Study the drawing (mm; zero at the part's minimum x, y, z) and answer. A direction names the side the tool comes from. Coordinates: 2 decimals unless noted, no trailing zeros. Order: outer loops, then holes, each group sorted by start corner. A loop starts at its lowest first (then second) coordinate and runs counter-clockwise, first axis right, second up. Notation, with made-up numbers: (62.25, -20.5) -> (108.25, -20.5) arc R29 ccw to (108.25, 15.5) -> close; hole circle Ø7 at (16, 29.5). An arc over 180 degrees is marked (long way). Put each result on its own line as item: value. Start each with the question number.
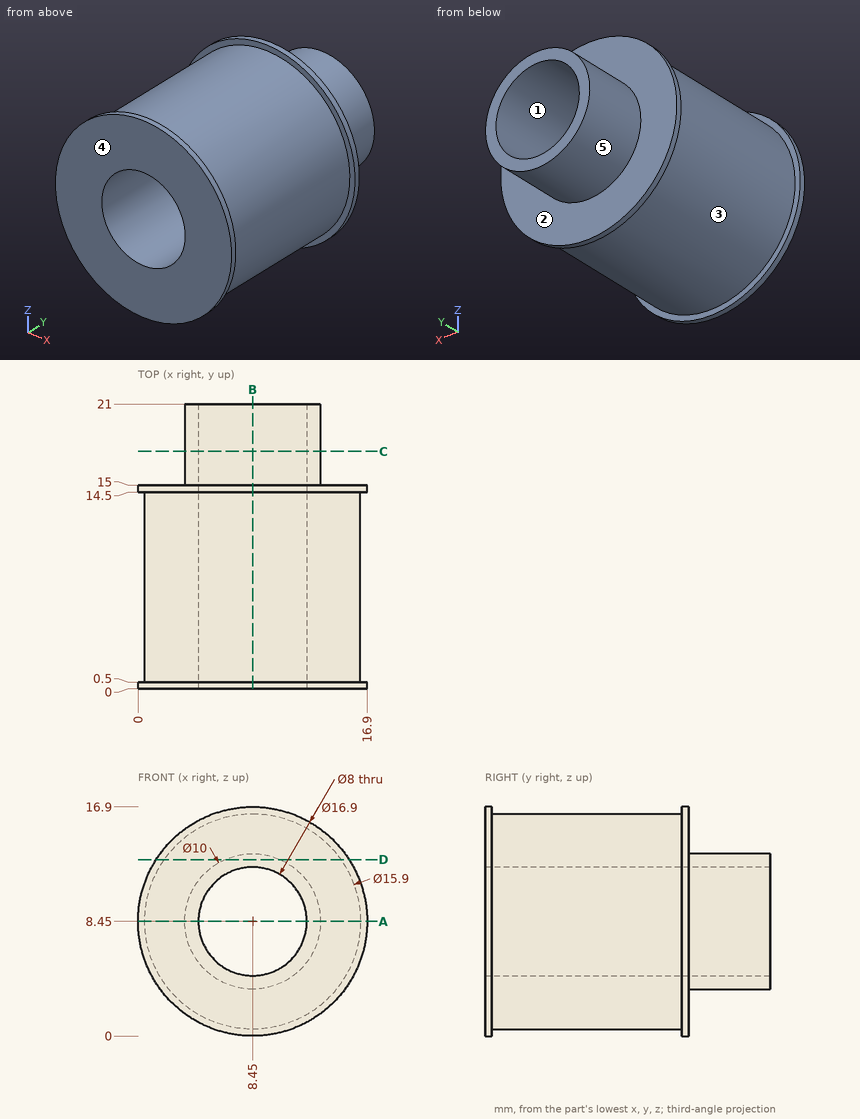
(1) The part is cut by section A-A on z = 8.45. Determine the outline of the cut face in (x, y).
(2) A tool of negligible diameter and unlimited length cuts with its end or side. For the marked faces 4 and 5, from which of +Z, -Z, +X, -X, +Y, -Y can it reach the whole face along a straight path? Write none if from no direction.
(3) For a pull along X with two mould halves and no side action, classify the marked faces 1, 2 and 3 as released by +X, released by -X, zero draft, split by the parting line, or undercut.
(4) The part is cut by section C-C on y = 17.5. Determine the outline of the cut face in (x, z).
(5) Each of these flat-tipped pins is pushed along its axis until it touches: P1, Ø3, axis at y = 6, z = 3.5, coming from the +X side; P2, Ø6, axis at x = 6, y = 7, coming from the +Z side; P3, Ø4, axis at y = 9, z = 5, coming from the +X side. Where does it stop, or does it pass through?
(6) Find the intervals of material crossed by L1, parallel to X at y = 9, z = 8.45; L2, parallel to X at y = 16, z = 8.45; L3, parallel to Y at x = 7.25, z = 2, in increasing order.
(7) The part is cut by section B-B on x = 8.45. Determine the outline of the cut face in (y, z), plus the area to 4 significant figures.
(8) The part is cut by section D-D on z = 13. Determine the outline of the cut face in (x, y).
Worked out:
1. outline: (0, 0) -> (4.45, 0) -> (4.45, 21) -> (3.45, 21) -> (3.45, 15) -> (0, 15) -> (0, 14.5) -> (0.5, 14.5) -> (0.5, 0.5) -> (0, 0.5) -> close; (12.45, 0) -> (16.9, 0) -> (16.9, 0.5) -> (16.4, 0.5) -> (16.4, 14.5) -> (16.9, 14.5) -> (16.9, 15) -> (13.45, 15) -> (13.45, 21) -> (12.45, 21) -> close
2. face 4: +Z, -Z, +X, -X, -Y
2. face 5: +Y
3. face 1: undercut
3. face 2: zero draft
3. face 3: split by the parting line
4. outline: circle Ø10 at (8.45, 8.45); hole circle Ø8 at (8.45, 8.45)
5. P1: x = 15.61
5. P2: z = 16.4
5. P3: x = 16.27
6. L1: 0.5 to 4.45, 12.45 to 16.4
6. L2: 3.45 to 4.45, 12.45 to 13.45
6. L3: 0 to 15
7. outline: (0, 0) -> (0.5, 0) -> (0.5, 0.5) -> (14.5, 0.5) -> (14.5, 0) -> (15, 0) -> (15, 3.45) -> (21, 3.45) -> (21, 4.45) -> (0, 4.45) -> close; (0, 12.45) -> (21, 12.45) -> (21, 13.45) -> (15, 13.45) -> (15, 16.9) -> (14.5, 16.9) -> (14.5, 16.4) -> (0.5, 16.4) -> (0.5, 16.9) -> (0, 16.9) -> close
7. area: 131.5 mm2
8. outline: (1.33, 0) -> (15.57, 0) -> (15.57, 0.5) -> (14.97, 0.5) -> (14.97, 14.5) -> (15.57, 14.5) -> (15.57, 15) -> (10.52, 15) -> (10.52, 21) -> (6.38, 21) -> (6.38, 15) -> (1.33, 15) -> (1.33, 14.5) -> (1.93, 14.5) -> (1.93, 0.5) -> (1.33, 0.5) -> close
